```python
from build123d import *

# Parameters (mm, degrees)
SKETCH_1_W          = 30
SKETCH_1_H          = 20
SKETCH_1_R          = 1.6
EXTRUDE_1_DEPTH     = 25
FILLET_1_R          = 3
SKETCH_2_R          = 1.6
CUT_EXTRUDE_1_DEPTH = 31
SKETCH_3_R          = 1.6
EXTRUDE_2_DEPTH     = 30
SKETCH_4_R          = 1.6
CUT_EXTRUDE_2_DEPTH = 31


with BuildPart() as part:
    # 草图1 → 凸台-拉伸1 (new body)
    with BuildSketch(Plane(origin=(0, 0, 0), x_dir=(1, 0, 0), z_dir=(0, 1, 0))):
        Rectangle(SKETCH_1_W, SKETCH_1_H)
        with Locations((-8, 7.5)):
            Circle(SKETCH_1_R, mode=Mode.SUBTRACT)
        with Locations((-8, -7.5)):
            Circle(SKETCH_1_R, mode=Mode.SUBTRACT)
        with Locations((8, -7.5)):
            Circle(SKETCH_1_R, mode=Mode.SUBTRACT)
        with Locations((8, 7.5)):
            Circle(SKETCH_1_R, mode=Mode.SUBTRACT)
    extrude(amount=EXTRUDE_1_DEPTH)

    # 圆角1
    fillet_1_edges = [part.edges().sort_by_distance(p)[0] for p in [
        (15, 12.5, 10),
        (-15, 12.5, 10),
        (-15, 12.5, -10),
        (15, 12.5, -10),
    ]]
    fillet(fillet_1_edges, radius=FILLET_1_R)

    # 草图2 → 切除-拉伸1 (cut, through all)
    with BuildSketch(Plane(origin=(15, 0, 0), x_dir=(0, 0, -1), z_dir=(1, 0, 0))):
        with Locations((0, 16.7)):
            Circle(SKETCH_2_R)
        with Locations((0, 8.3)):
            Circle(SKETCH_2_R)
    extrude(amount=-CUT_EXTRUDE_1_DEPTH, mode=Mode.SUBTRACT)

    # 草图3 → 凸台-拉伸2 (add)
    with BuildSketch(Plane(origin=(15, 0, 0), x_dir=(0, 0, -1), z_dir=(1, 0, 0))):
        with Locations((0, 16.7)):
            Circle(SKETCH_3_R)
    extrude(amount=-EXTRUDE_2_DEPTH)

    # 草图4 → 切除-拉伸2 (cut, through all)
    with BuildSketch(Plane(origin=(15, 0, 0), x_dir=(0, 0, -1), z_dir=(1, 0, 0))):
        with Locations((0, 16.7)):
            Circle(SKETCH_4_R)
    extrude(amount=-CUT_EXTRUDE_2_DEPTH, mode=Mode.SUBTRACT)


solid = part.part
```
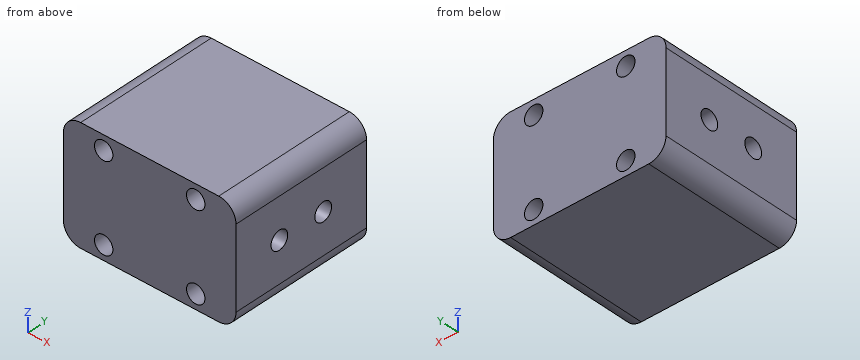
Can you work these out from the model? Positions are in its coordinate system, mm. Coordinates: 2 decimals unless noted, no trailing zeros. Order: outer loops, then holes, each group sorted by start corner. A loop starts at its lowest first (then second) coordinate and runs counter-clockwise, first axis right, second up.
1. If we section it at B-B (y = 16.7): Please give me the cut outline in (x, z), then the cut area to 3 significant figures.
2. If we section it at A-A (x = -8): Please give me the cut outline in (y, z), then the cut area to 3 significant figures.
3. If we section it at D-D (z = -6.5): Please give me the cut outline in (x, y).
4. If we section it at C-C (x = 0.5): Please give me the cut outline in (y, z).
5. I need wall thicknesses on line 1 (Y direction, x = -5.5, z = 0); line 2 (X direction, y = 13.5, z = 7.25); line 3 (Z direction, x = 8, y = 13.5). Which ranges of each line are inside material? Lowest first, please.
Entries:
1. outline: (-15, -7) arc R3 ccw to (-12, -10) - (12, -10) arc R3 ccw to (15, -7) - (15, -1.6) - (-15, -1.6) - close; (-15, 1.6) - (15, 1.6) - (15, 7) arc R3 ccw to (12, 10) - (-12, 10) arc R3 ccw to (-15, 7) - close; hole circle Ø3.2 at (-8, -7.5); hole circle Ø3.2 at (-8, 7.5); hole circle Ø3.2 at (8, -7.5); hole circle Ø3.2 at (8, 7.5)
1. area: 464 mm2
2. outline: (0, -10) - (25, -10) - (25, -9.1) - (0, -9.1) - close; (0, -5.9) - (25, -5.9) - (25, 5.9) - (0, 5.9) - close; (0, 9.1) - (25, 9.1) - (25, 10) - (0, 10) - close; hole circle Ø3.2 at (8.3, 0); hole circle Ø3.2 at (16.7, 0)
2. area: 324 mm2
3. outline: (-15, 0) - (-9.25, 0) - (-9.25, 25) - (-15, 25) - close; (-6.75, 0) - (6.75, 0) - (6.75, 25) - (-6.75, 25) - close; (9.25, 0) - (15, 0) - (15, 25) - (9.25, 25) - close
4. outline: (0, -10) - (25, -10) - (25, 10) - (0, 10) - close; hole circle Ø3.2 at (8.3, 0); hole circle Ø3.2 at (16.7, 0)
5. line 1: y = 0 to 6.7, 9.9 to 15.1, 18.3 to 25
5. line 2: x = -14.99 to -9.58, -6.42 to 6.42, 9.58 to 14.99
5. line 3: z = -10 to -9.1, -5.9 to 5.9, 9.1 to 10
